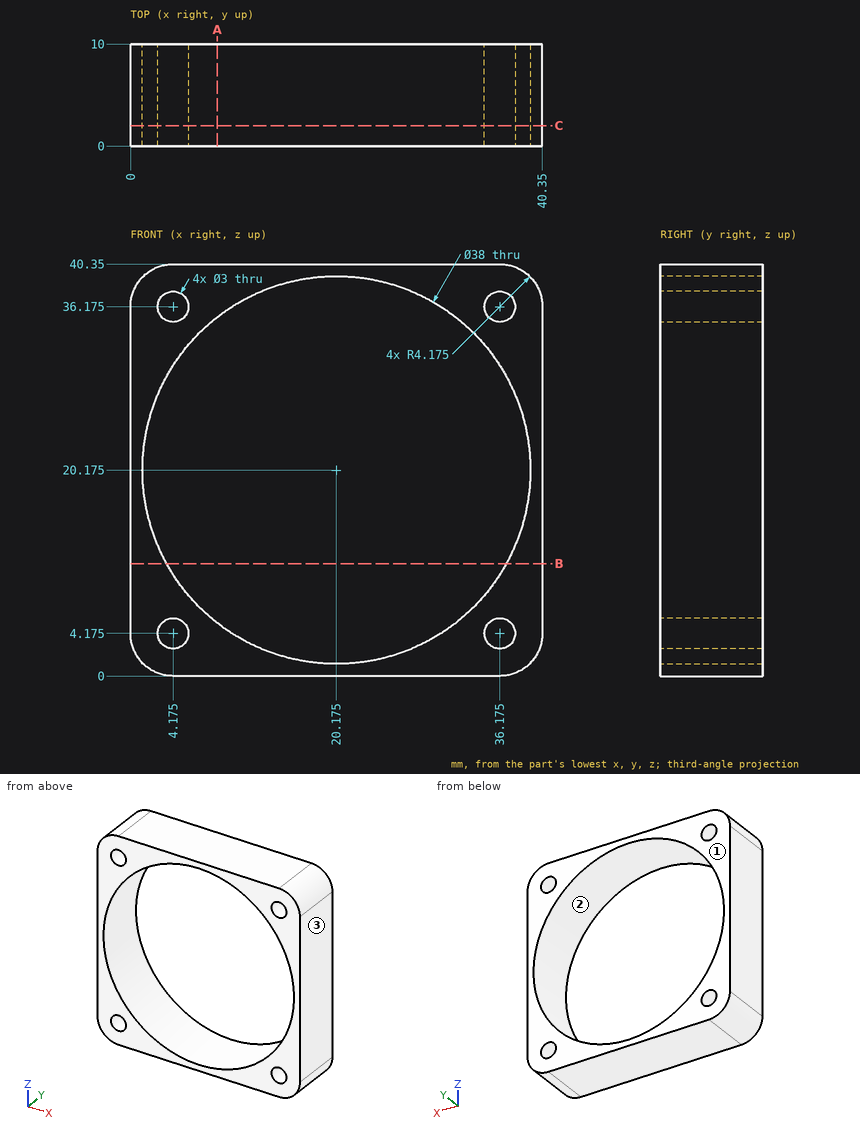
Drawing for the job (mm, zero at the part's lowest x, y, z). Coordinates: 2 decimals unless noted, no trailing zeros. Order: outer loops, then holes, each group sorted by start corner. A loop starts at its lowest first (then second) coordinate and runs counter-clockwise, first axis right, second up.
Item 1: Band-saw the part on A-A on x = 8.5. List the corners of the cut face in (y, z), plus the area to 3 significant figures.
Check sheet entries:
outline: (0, 0) - (10, 0) - (10, 5.19) - (0, 5.19) - close; (0, 35.16) - (10, 35.16) - (10, 40.35) - (0, 40.35) - close
area: 104 mm2
Item 2: Band-saw the part on B-B on z = 11. List the corners of the cut face in (x, y), plus the area to 3 significant figures.
Check sheet entries:
outline: (0, 0) - (3.54, 0) - (3.54, 10) - (0, 10) - close; (36.81, 0) - (40.35, 0) - (40.35, 10) - (36.81, 10) - close
area: 70.7 mm2
Item 3: Band-saw the part on C-C on y = 2. List the corners of the cut face in (x, z) (3 decimals).
Check sheet entries:
outline: (0, 4.175) arc R4.175 ccw to (4.175, 0) - (36.175, 0) arc R4.175 ccw to (40.35, 4.175) - (40.35, 36.175) arc R4.175 ccw to (36.175, 40.35) - (4.175, 40.35) arc R4.175 ccw to (0, 36.175) - close; hole circle Ø38 at (20.175, 20.175); hole circle Ø3 at (4.175, 4.175); hole circle Ø3 at (4.175, 36.175); hole circle Ø3 at (36.175, 4.175); hole circle Ø3 at (36.175, 36.175)
Item 4: Drill centre lines: L1, parallel to X at y = 9, z = 4.5; L2, parallel to X at y = 4.5, z = 3. Where is each one in solid material? Low to high.
Check sheet entries:
L1: x = 0 to 2.71, 5.64 to 9.44, 30.91 to 34.71, 37.64 to 40.35
L2: x = 0.17 to 3.24, 5.11 to 12.05, 28.3 to 35.24, 37.11 to 40.18
Item 5: Two-plate mould, pull along X, no slides. Class the marked faces 1, 2 and 3: +X half, -X half, draft (parallel to the pull), parting line (faces both ways), or undercut.
Check sheet entries:
face 1: draft
face 2: undercut
face 3: +X half
